```python
from build123d import *

# Parameters (mm, degrees)
SKETCH1_W           = 9.8
SKETCH1_H           = 8.9
SKETCH1_R           = 1
BOSS_EXTRUDE2_DEPTH = 3
BOSS_EXTRUDE4_DEPTH = 10
SKETCH4_R           = 1.925
BOSS_EXTRUDE5_DEPTH = 116
CUT_EXTRUDE1_START  = -2
CUT_EXTRUDE1_DEPTH  = 2
BOSS_EXTRUDE6_REACH = 122.306
SKETCH9_R           = 1.925


with BuildPart() as part:
    # Sketch1 → Boss-Extrude2 (new body)
    with BuildSketch(Plane.XY):
        Rectangle(SKETCH1_W, SKETCH1_H)
        with Locations((0, -2.95)):
            Circle(SKETCH1_R, mode=Mode.SUBTRACT)
    extrude(amount=BOSS_EXTRUDE2_DEPTH)

    # Sketch3 → Boss-Extrude4 (add)
    with BuildSketch(Plane(origin=(0, 4.45, 0), x_dir=(1, 0, 0), z_dir=(0, 1, 0))):
        with BuildLine():
            Line((4.9, -3), (4.9, 0))
            Line((4.9, 0), (4.242640687, 0))
            ThreePointArc((4.242640687, 0), (0, 3), (-4.242640687, 0))
            Line((-4.242640687, 0), (-4.9, 0))
            Line((-4.9, 0), (-4.9, -3))
            Line((-4.9, -3), (-4.242640687, -3))
            ThreePointArc((-4.242640687, -3), (0, -6), (4.242640687, -3))
            Line((4.242640687, -3), (4.9, -3))
        make_face()
    extrude(amount=BOSS_EXTRUDE4_DEPTH)

    # Sketch4 → Boss-Extrude5 (add)
    with BuildSketch(Plane(origin=(0, 14.45, 0), x_dir=(1, 0, 0), z_dir=(0, 1, 0))):
        with Locations(Location((0, -1.5, 0), (0, 0, 90))):
            Circle(SKETCH4_R)
    extrude(amount=BOSS_EXTRUDE5_DEPTH)

    # Sketch7 → Revolve1 (revolve)
    with BuildSketch(Plane.XY.offset(1.5)):
        with BuildLine():
            Line((3.230940108, 123.05), (6.92598183, 129.45))
            ThreePointArc((6.92598183, 129.45), (7.658032638, 130.182050808), (8.658032638, 130.45))
            Line((8.658032638, 130.45), (17.5, 130.45))
            Line((17.5, 130.45), (17.5, 131.95))
            Line((17.5, 131.95), (0, 131.95))
            Line((0, 131.95), (0, 130.45))
            Line((0, 130.45), (1.925, 130.45))
            Line((1.925, 130.45), (1.925, 122.65))
            Line((1.925, 122.65), (2.538119785, 122.65))
            ThreePointArc((2.538119785, 122.65), (2.938119785, 122.757179677), (3.230940108, 123.05))
        make_face()
    revolve(axis=Axis((0, 130.45, 1.5), (0, 1, 0)))

    # Sketch8 → Cut-Extrude1 (cut)
    with BuildSketch(Plane(origin=(0, 14.45, 0), x_dir=(1, 0, 0), z_dir=(0, 1, 0)).offset(CUT_EXTRUDE1_START)):
        with BuildLine():
            Line((-4.242640687, 0), (-4.9, 0))
            Line((-4.9, 0), (-4.9, -3))
            Line((-4.9, -3), (-4.242640687, -3))
            ThreePointArc((-4.242640687, -3), (0, -6), (4.242640687, -3))
            Line((4.242640687, -3), (4.9, -3))
            Line((4.9, -3), (4.9, 0))
            Line((4.9, 0), (4.242640687, 0))
            ThreePointArc((4.242640687, 0), (0, 3), (-4.242640687, 0))
        make_face()
    extrude(amount=CUT_EXTRUDE1_DEPTH, mode=Mode.SUBTRACT)


with BuildPart() as cut_extrude1_piece_1:
    # of the separate pieces the step leaves, piece 1, a body of its own (cut_extrude1_pieces)
    add(part.part.solids().sort_by_distance((0, 14.45, -0.425))[0])


with BuildPart() as cut_extrude1_piece_2:
    # of the separate pieces the step leaves, piece 2, a body of its own (cut_extrude1_pieces)
    add(part.part.solids().sort_by_distance((4.9, -4.45, 0))[0])

    # Sketch9 → Boss-Extrude6 (add, up to next)
    with BuildSketch(Plane.XZ.offset(-14.45), mode=Mode.PRIVATE) as boss_extrude6_sk1:
        with Locations(Location((0, 1.5, 0), (0, 0, 270))):
            Circle(SKETCH9_R)
    boss_extrude6_tool1 = extrude(boss_extrude6_sk1.sketch, amount=BOSS_EXTRUDE6_REACH, mode=Mode.PRIVATE) - cut_extrude1_piece_2.part

    add(cut_extrude1_piece_1.part)  # Boss-Extrude6 merges Cut-Extrude1 piece 1
    add(boss_extrude6_tool1.solids().sort_by_distance((0, 14.45, 1.5))[0])


solid = cut_extrude1_piece_2.part
```
Check sheet for the modelled part. Datum: model origin and axes. Units: mm. A direction names the side the tool comes from. Round coordinates to 2 decimals unless told otherwise and drop trailing zeros. Order: outer loops, then holes, each group sorted by start corner. A loop starts at its lowest first (then second) coordinate and runs counter-clockwise, first axis right, second up. Notation, with made-up numbers: M 76,29.25 L 93,29.25 A20 cw 93,53.25 Z; hole C 19.25,40 d6. An arc over 180 degrees is marked long. Answer in a Markdown table with one row per item.
(1) Section check A-A on z = 1.5. Record the boundary of the cut face in (x, y) (3 decimals), plus the area to 3 significant figures.
Findings:
| item | result |
|---|---|
| outline | M -17.5,130.45 L -8.658,130.45 A2 cw -6.926,129.45 L -3.231,123.05 A0.8 ccw -2.538,122.65 L -1.925,122.65 L -1.925,12.45 L -4.9,12.45 L -4.9,-4.45 L 4.9,-4.45 L 4.9,12.45 L 1.925,12.45 L 1.925,122.65 L 2.538,122.65 A0.8 ccw 3.231,123.05 L 6.926,129.45 A2 cw 8.658,130.45 L 17.5,130.45 L 17.5,131.95 L -17.5,131.95 Z; hole C 0,-2.95 d2 |
| area | 722 mm^2 |
(2) Section check B-B on y = 22. Record the boundary of the cut face in (x, z) (3 decimals), plus the area to 3 significant figures.
Findings:
| item | result |
|---|---|
| outline | C 0,1.5 d3.85 |
| area | 11.6 mm^2 |
(3) Section check D-D on z = -10.5. Record the boundary of the cut face in (x, y).
Findings:
| item | result |
|---|---|
| outline | M -12.74,130.45 L 12.74,130.45 L 12.74,131.95 L -12.74,131.95 Z |
(4) Draft check along Y on faces 5 (the flat face through (0, 4.45, 4)), 6 (the cylindrical face through (0.578, 68.321, -0.336)), 7 (the flat face through (0, 2, 3)). Enter one of: +Y half, -Y half, draft (parallel to the pull), parting line (faces both ways), or undercut.
Findings:
| item | result |
|---|---|
| face 5 | -Y half |
| face 6 | undercut |
| face 7 | draft |
(5) Gauge pin test, flat ends, axial feed: pin 1 (2.5 mm diameter, centred on x = 0, y = -2.95, fed in from -Z); pin 2 (2 mm diameter, centred on x = 1.5, y = 70, fed in from -Z); pin 3 (1.5 mm diameter, centred on x = -2, z = 4, fed in from -Y); pin 4 (2.5 mm diameter, centred on x = 0.5, z = 4, fed in from -Y). Record the tip position at first contact, or that the pin passes through.
Findings:
| item | result |
|---|---|
| pin 1 | stops at z = 0 |
| pin 2 | stops at z = -0.36 |
| pin 3 | stops at y = 4.45 |
| pin 4 | stops at y = -4.45 |
(6) Material ranges on line 1 along Y through (x, z) = (0, 1); line 2 along Y through (x, z) = (-10.5, 4.5); line 3 along Y through (x, z) = (-3, 1), recorded low to high. Write a range as from..to.
Findings:
| item | result |
|---|---|
| line 1 | y = -4.45..-3.95, -1.95..131.95 |
| line 2 | y = 130.45..131.95 |
| line 3 | y = -4.45..12.45, 122.83..131.95 |
(7) Set-up check for faces 1 (the flat face through (8.023, 130.45, 5.144)), 2 (the conical face through (3.694, 124.161, 0.337)), 3 (the cylindrical face through (0, 8, -3)), 4 (the cylindrical face through (0, 8, 6)): record each of +Z, -Z, +X, -X, +Y, -Y from which the full face is reachable in a straight line by a thin tool's end or side.
Findings:
| item | result |
|---|---|
| face 1 | -Y |
| face 2 | none |
| face 3 | -Z, -Y |
| face 4 | +Z, -Y |
(8) Section check C-C on x = -10. Record the boundary of the cut face in (y, z), plus the area to 3 significant figures.
Findings:
| item | result |
|---|---|
| outline | M 130.45,-12.86 L 131.95,-12.86 L 131.95,15.86 L 130.45,15.86 Z |
| area | 43.1 mm^2 |
